Check sheet for the modelled part. Datum: model origin and axes. Units: mm. A direction names the side the tool comes from. Coordinates: 2 decimals unless noted, no trailing zeros. Write each loop counter-clockwise with the first axis right and the second up, starting at its lowest first coordinate (ties: lowest second). Pieces come first, ordered by that corner, then holes. Notation, with made-up numbers: M 70.5,5.5 L 128.5,5.5 A31 ccw 128.5,42.5 Z; hole C 33.5,63 d1. An arc over 180 degrees is marked long. Answer as CSV lines item,"result". Start each with the question number.
1) Section check D-D (z = -4.25). Record the cut outline in (x, y), and give its area (3 significant figures).
2) Draft check along X on faces 4 (the flat face through (9.801, 4, 5)), 5 (the flat face through (0, 1, -13.15)), 6 (the flat face through (-24.782, 3, 5)), 7 (the flat face through (12.709, 2, 5)). Enter one of: +X half, -X half, draft (parallel to the pull), parting line (faces both ways), or undercut.
3) Material ranges on L1, parallel to X at y = 3.5, z = 11.5; L2, parallel to X at y = 4.5, z = 3.75; L3, parallel to Y at x = 27.5, z = -3.5, recorded low to high. Write a range as [from, to].
4) Section check C-C (x = -6.5). Record the cut outline in (y, z).
5) Section check B-B (z = 0.5). Record the cut outline in (x, y), and give its area (3 significant figures).
6) Section check A-A (y = 4.25). Record the cut outline in (x, z).
7) Go/stop test with flat-tipped pins: pin 1 Ø8 at (x, z) = (15.5, -3.5) entering from +Y; pin 2 Ø2 at (y, z) = (4, 11) entering from -X; pin 3 Ø1.4 at (y, z) = (3, -9) entering from +X. Record where each tip stops, or that it passes through.
8) Access from +Z, -Z, +X, -X, +Y, -Y to the whole of each face (thin tool, end or side, straight path). Record for faces 1 (the flat face through (-24, 3, 12.654)), 2 (the flat face through (-11.144, 2, 1)), 3 (the flat face through (-22.367, 3, -9)).
Autodesk Inventor part; units mm, degrees
ref_plane "YZ Plane" through (0, 0, 0) normal (1, 0, 0) x (0, 1, 0)
ref_plane "XZ Plane" through (0, 0, 0) normal (0, 1, 0) x (-1, 0, 0)
ref_plane "XY Plane" through (0, 0, 0) normal (0, 0, 1) x (1, 0, 0)
sketch "Boceto1" plane through (0, 0, 0) normal (0, 1, 0) x (-1, 0, 0)
  line L0 (-25, 13.15) -> (25, 13.15)
  line L1 (25, 13.15) -> (25, -13.15)
  line L2 (25, -13.15) -> (-25, -13.15)
  line L3 (-25, -13.15) -> (-25, 13.15)
  line L4 (-25, 13.15) -> (25, -13.15) construction
  line L5 (25, 13.15) -> (-25, -13.15) construction
  point P0 (0, 0)
  dimension "d0" = 50
  dimension "d1" = 26.3
extrude "Extrusión1" add sketch "Boceto1" along normal blind 1.6
sketch "Boceto2" plane through (0, 1.6, 0) normal (0, 1, 0) x (1, 0, 0)
  line L0 (15.6711, -6.5623) -> (32.2824, -6.5623)
  line L1 (32.2824, -6.5623) -> (32.2824, 6.5623)
  line L2 (32.2824, 6.5623) -> (15.6711, 6.5623)
  line L3 (15.6711, 6.5623) -> (15.6711, -6.5623)
  line L4 (15.6711, -6.5623) -> (32.2824, 6.5623) construction
  line L5 (32.2824, -6.5623) -> (15.6711, 6.5623) construction
  point P0 (0, 0)
  point P1 (23.9767, 0)
extrude "Extrusión2" add sketch "Boceto2" along normal blind 0.5
sketch "Boceto3" plane through (0, 2.1, 0) normal (0, 1, 0) x (1, 0, 0)
  line L0 (24.9953, -5.8962) -> (16.4546, -5.8962)
  line L1 (16.4546, -5.8962) -> (16.4546, 5.8962)
  line L2 (16.4546, 5.8962) -> (24.9953, 5.8962)
  line L3 (24.9953, 5.8962) -> (24.9953, -5.8962)
  line L4 (24.9953, -5.8962) -> (16.4546, 5.8962) construction
  line L5 (16.4546, -5.8962) -> (24.9953, 5.8962) construction
  point P0 (0, 0)
  point P1 (20.725, 0)
extrude "Extrusión3" add sketch "Boceto3" along normal blind 1.5
sketch "Boceto4" plane through (0, 1.6, 0) normal (0, 1, 0) x (1, 0, 0)
  line L0 (-24.7819, -12.6535) -> (-22.3667, -12.6535)
  line L1 (-22.3667, -12.6535) -> (-22.3667, 3.0977)
  line L2 (-22.3667, 3.0977) -> (-24.7819, 3.0977)
  line L3 (-24.7819, 3.0977) -> (-24.7819, -12.6535)
  line L4 (-24.7819, 5.6879) -> (-22.3667, 5.6879)
  line L5 (-22.3667, 5.6879) -> (-22.3667, 12.3034)
  line L6 (-22.3667, 12.3034) -> (-24.7819, 12.3034)
  line L7 (-24.7819, 12.3034) -> (-24.7819, 5.6879)
  line L8 (-18.3064, -12.6535) -> (-7.2456, -12.6535)
  line L9 (-7.2456, -12.6535) -> (-7.2456, -10.0983)
  line L10 (-7.2456, -10.0983) -> (-18.3064, -10.0983)
  line L11 (-18.3064, -10.0983) -> (-18.3064, -12.6535)
  line L12 (-7.2456, -12.6535) -> (-3.8465, -12.6535)
  line L13 (-3.8465, -12.6535) -> (-3.8465, -10.0983)
  line L14 (-3.8465, -10.0983) -> (-7.2456, -10.0983)
  line L15 (-7.2456, -10.0983) -> (-7.2456, -12.6535)
  point P0 (0, 0)
extrude "Extrusión4" add sketch "Boceto4" along normal blind 3.7
sketch "Boceto5" plane through (0, 1.6, 0) normal (0, 1, 0) x (1, 0, 0)
  line L0 (9.1061, -9.0184) -> (12.7089, -9.0184)
  line L1 (12.7089, -9.0184) -> (12.7089, -1.3991)
  line L2 (12.7089, -1.3991) -> (9.1061, -1.3991)
  line L3 (9.1061, -1.3991) -> (9.1061, -9.0184)
  line L4 (-11.1445, -3.83) -> (-2.9401, -3.83)
  line L5 (-2.9401, -3.83) -> (-2.9401, 2.5512)
  line L6 (-2.9401, 2.5512) -> (-11.1445, 2.5512)
  line L7 (-11.1445, 2.5512) -> (-11.1445, -3.83)
  point P0 (0, 0)
extrude "Extrusión5" add sketch "Boceto5" along normal blind 1
sketch "Boceto6" plane through (0, 1.6, 0) normal (0, 1, 0) x (1, 0, 0)
  line L0 (-14.2306, 5.4877) -> (-10.7922, 5.4877)
  line L1 (-10.7922, 5.4877) -> (-10.7922, 11.4752)
  line L2 (-10.7922, 11.4752) -> (-14.2306, 11.4752)
  line L3 (-14.2306, 11.4752) -> (-14.2306, 5.4877)
  point P0 (0, 0)
extrude "Extrusión6" add sketch "Boceto6" along normal blind 4.7
sketch "Boceto7" plane through (0, 2.6, 0) normal (0, 1, 0) x (1, 0, 0)
  line L0 (9.8007, -8.1731) -> (12.0409, -8.1731)
  line L1 (12.0409, -8.1731) -> (12.0409, -2.1527)
  line L2 (12.0409, -2.1527) -> (9.8007, -2.1527)
  line L3 (9.8007, -2.1527) -> (9.8007, -8.1731)
  point P0 (0, 0)
extrude "Extrusión7" add sketch "Boceto7" along normal blind 3.7
sketch "Boceto8" plane through (0, 0, 0) normal (0, -1, 0) x (1, 0, 0)
  line L0 (-25, -13.15) -> (-25, 13.15)
  line L1 (-25, 0) -> (-22.5, 0)
  line L2 (-22.5, 0) -> (-22.5, -12.5)
  line L3 (-22.5, -12.5) -> (-14.5, -12.5)
  line L4 (-24.7819, -12.3034) -> (-22.3667, -12.3034)
  line L5 (-22.5, -12.5) -> (-14.5, -12.5) construction
  line L6 (-14.5, -12.5) -> (-14.5, 12.5)
  line L7 (-14.5, 12.5) -> (-22.5, 12.5)
  line L8 (-25, 13.15) -> (25, 13.15)
  line L9 (-22.5, 12.5) -> (-22.5, 0)
  point P0 (0, 0)
  dimension "d16" = 2.5
  dimension "d17" = 12.5
  dimension "d18" = 8
  dimension "d19" = 0
  dimension "d20" = 25
extrude "Extrusión8" add sketch "Boceto8" along normal blind 5.7
properties part number "Nordic_PCB"
Results found:
1,outline,"M -25,0 L -22.5,0 L -22.5,-5.7 L -14.5,-5.7 L -14.5,0 L 25,0 L 25,1.6 L 32.28,1.6 L 32.28,2.1 L 25,2.1 L 25,3.6 L 16.45,3.6 L 16.45,2.1 L 15.67,2.1 L 15.67,1.6 L -25,1.6 Z"
1,area,"147 mm2"
2,face 4,"undercut"
2,face 5,"draft"
2,face 6,"-X half"
2,face 7,"undercut"
3,L1,"x = [-24.78, -22.37], [-18.31, -3.85]"
3,L2,"x = [-24.78, -22.37], [9.8, 12.04]"
3,L3,"y = [1.6, 2.1]"
4,outline,"M 0,-13.15 L 1.6,-13.15 L 1.6,-2.55 L 2.6,-2.55 L 2.6,3.83 L 1.6,3.83 L 1.6,10.1 L 5.3,10.1 L 5.3,12.65 L 1.6,12.65 L 1.6,13.15 L 0,13.15 Z"
5,outline,"M -25,0 L -22.5,0 L -22.5,-5.7 L -14.5,-5.7 L -14.5,0 L 25,0 L 25,1.6 L 32.28,1.6 L 32.28,2.1 L 25,2.1 L 25,3.6 L 16.45,3.6 L 16.45,2.1 L 15.67,2.1 L 15.67,1.6 L -2.94,1.6 L -2.94,2.6 L -11.14,2.6 L -11.14,1.6 L -22.37,1.6 L -22.37,5.3 L -24.78,5.3 L -24.78,1.6 L -25,1.6 Z"
5,area,"164 mm2"
6,outline,"M -24.78,-12.3 L -22.37,-12.3 L -22.37,-5.69 L -24.78,-5.69 Z; M -24.78,-3.1 L -22.37,-3.1 L -22.37,12.65 L -24.78,12.65 Z; M -18.31,10.1 L -3.85,10.1 L -3.85,12.65 L -18.31,12.65 Z; M -14.23,-11.48 L -10.79,-11.48 L -10.79,-5.49 L -14.23,-5.49 Z; M 9.8,2.15 L 12.04,2.15 L 12.04,8.17 L 9.8,8.17 Z"
7,pin 1,"stops at y = 3.6"
7,pin 2,"stops at x = -24.78"
7,pin 3,"stops at x = -10.79"
8,face 1,"+Z, +X, -X, +Y"
8,face 2,"+Y"
8,face 3,"+Z, -Z, +Y"
